```python
from build123d import *

# Parameters (mm, degrees)
F0_R     = 22.225
F0_R_2   = 6.35
F1_DEPTH = 3.175


# Not quite as in the source:
# - a feature names something its author has since deleted; it is built from what else it names


with BuildPart() as f1:
    # F0 (on Top) → F1 (new body)
    with BuildSketch(Plane.XY):
        Polygon((-217.8399659125, 274.6944633329), (-274.3403279131, 274.6944633329), (-249.4802269343, 223.6304721332), (-194.8479709943, 227.4676629604), align=None)
        with Locations((-233.2169740796, 248.1006040146)):
            Circle(F0_R, mode=Mode.SUBTRACT)
        with Locations((-233.2169740796, 248.1006040146)):
            Circle(F0_R)
        with Locations((-233.2169740796, 248.1006040146)):
            Circle(F0_R_2, mode=Mode.SUBTRACT)
        Polygon((-274.3403279131, 314.3819633329), (-274.3403279131, 274.6944633329), (-217.8399659125, 274.6944633329), (-233.0653279131, 305.9681798747), (-233.0653279131, 314.3819633329), align=None)
        Polygon((-233.0653279131, 305.9681798747), (-217.8399659125, 274.6944633329), (215.3278746861, 274.6944633329), (284.0686411115, 314.3819633329), (-233.0653279131, 314.3819633329), align=None)
        Polygon((215.3278746861, 274.6944633329), (-217.8399659125, 274.6944633329), (-194.8479709943, 227.4676629604), (179.0097919037, 253.726208462), align=None)
    extrude(amount=F1_DEPTH)


solid = f1.part
```
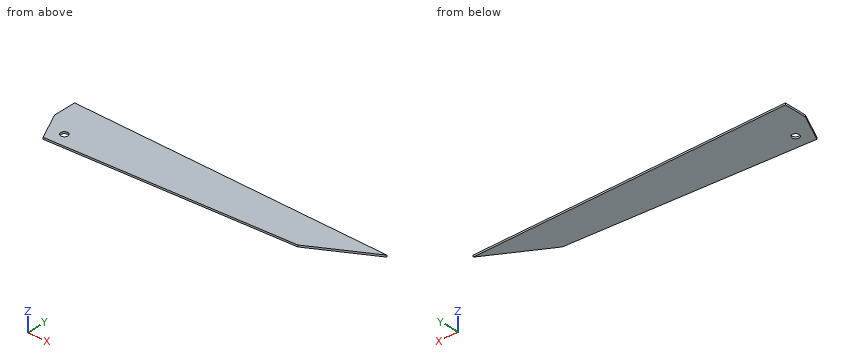
Source: CAD feature listing. Evaluate the final solid. Frame: model axes, mm. Give positions to 0.01 mm unless a question says otherwise; leave off trailing zeros. Loops run counter-clockwise (first coordinate to the right, second up) from the corner with the lowest first, then second, coordinate; pieces in that order, holes last. Notation, with made-up numbers: (-12, 12) - (38, 12) arc R22 cw to (38, 35) - close; hole circle Ø8 at (-29, -23.75). An arc over 180 degrees is marked (long way). Use CSV: the item, a comma, the result in double quotes.
1) Cut plane A-A (z = 0.5). Output: boundary loops of the cut face in (x, y).
Worked out:
outline,"(-274.34, 274.69) - (-249.48, 223.63) - (179.01, 253.73) - (284.07, 314.38) - (-274.34, 314.38) - close; hole circle Ø12.7 at (-233.22, 248.1)"
2) Cut plane C-C (x = -152.5). Output: boundary loops of the cut face in (y, z) (3 decimals), and give its area (3 significant figures).
Worked out:
outline,"(230.442, 0) - (314.382, 0) - (314.382, 3.175) - (230.442, 3.175) - close"
area,"267 mm^2"
3) Cut plane B-B (y = 233). Output: boundary loops of the cut face in (x, z) (3 decimals), and give its area (3 significant figures).
Worked out:
outline,"(-254.042, 0) - (-116.081, 0) - (-116.081, 3.175) - (-254.042, 3.175) - close"
area,"438 mm^2"
4) Line query: line 1 (Y direction, x = 109.5, z = 2.8); line 2 (Y direction, x = -8, z = 2.15); line 3 (X direction, y = 295.5, z = 0.9). Output: solid intervals per line, ascending.
Worked out:
line 1,"y = 248.84 to 314.38"
line 2,"y = 240.59 to 314.38"
line 3,"x = -274.34 to 251.36"
